from build123d import *

# Parameters (mm, degrees)
SKETCH1_W     = 3
SKETCH1_H     = 35
CHAMFER1_SIZE = 0.5


with BuildPart() as part:
    # Sketch1 → Revolve1 (revolve)
    with BuildSketch(Plane.XY):
        with Locations((1.5, 17.5)):
            Rectangle(SKETCH1_W, SKETCH1_H)
    revolve(axis=Axis((0, 0, 0), (0, 1, 0)))

    # Sketch3 → Groove for DIN 471 - 4 x 0.4, Circlip for shafts - normal1 (revolve, cut)
    with BuildSketch(Plane(origin=(0, 0, 0), x_dir=(0, 0, -1), z_dir=(-1, 0, 0))):
        with BuildLine():
            Line((2.55, -34.24), (3.6, -34.24))
            Line((3.6, -34.24), (3.6, -33.5))
            Line((3.6, -33.5), (2.55, -33.5))
            ThreePointArc((2.55, -33.5), (2.514644661, -33.514644661), (2.5, -33.55))
            Line((2.5, -33.55), (2.5, -34.19))
            ThreePointArc((2.5, -34.19), (2.514644661, -34.225355339), (2.55, -34.24))
        make_face()
    revolve(axis=Axis((0, 50, 0), (0, -1, 0)), mode=Mode.SUBTRACT)

    # Chamfer1
    chamfer1_edges = [part.edges().sort_by_distance(p)[0] for p in [
        (-3, 0, 0),
        (-3, 35, 0),
    ]]
    chamfer(chamfer1_edges, length=CHAMFER1_SIZE)


solid = part.part
CAD build for the part. Positions are in the model's coordinates, mm. A direction names the side the tool comes from. Round coordinates to 2 decimals unless told otherwise and drop trailing zeros. Write each loop counter-clockwise with the first axis right and the second up, starting at its lowest first coordinate (ties: lowest second). Pieces come first, ordered by that corner, then holes. Notation, with made-up numbers: M 29,79.25 L 84,79.25 A22 cw 84,85.25 Z; hole C 24,-31.75 d1. An arc over 180 degrees is marked long. Put each result on its own line as item: value. Start each with the question number.
1) Drill centre lines: probe 1 along Z at (x, y) = (-0.1, 32); probe 2 along X at (y, z) = (9, -1.65); probe 3 along Y at (x, z) = (2.55, -0.5). Where is each one in solid material? Low to high. Write a range as [from, to].
2) 3-axis set-ups, long thin cutter, end or side, ignore diameter. For faces 4 (the flat face through (0, 35, 0)), 5 (the cylindrical face through (-2.44, 33.87, 0.54)): which of +Z, -Z, +X, -X, +Y, -Y reach the whole face in a straight line?
3) Saw through at A-A, the plane y = 18.5. Write the cut outline in (x, z), and give its area (3 significant figures).
4) Pull direction Y, two halves, no side cores. Call faces 1 (the flat face through (2, 33.5, 2)), 2 (the flat face through (0, 0, 0)), 3 (the cylindrical face through (-3, 17, 0)): pulls with the +Y half, pulls with the -Y half, needs draft (parallel to the pull), parting line crosses it, or undercut.
5) Pin check, flat tip, straight feed: pin 1 Ø3 at (y, z) = (14, 2.5) entering from -X. Stop position of the tip, or through.
Resolved:
1. probe 1: [-3, 3]
1. probe 2: [-2.51, 2.51]
1. probe 3: [0.1, 33.5], [34.24, 34.9]
2. face 4: +Z, -Z, +X, -X, +Y
2. face 5: none
3. outline: C 0,0 d6
3. area: 28.3 mm²
4. face 1: undercut
4. face 2: pulls with the -Y half
4. face 3: needs draft
5. pin 1: x = -2.83
